CAD build for the part. Positions are in the model's coordinates, mm. A direction names the side the tool comes from. Give positions to 0.01 mm unless a question says otherwise; leave off trailing zeros. Loops run counter-clockwise (first coordinate to the right, second up) from the corner with the lowest first, then second, coordinate; pieces in that order, holes last. Notation, with made-up numbers: (88, 77) -> (131, 77) arc R22 cw to (131, 100) -> close; hole circle Ø2 at (15, 46.25). An arc over 180 degrees is marked (long way). Use one line per item in the form item = value.
```python
from build123d import *

# Parameters (mm, degrees)
SKETCH013_W     = 125.6
SKETCH013_H     = 46.6
PAD007_DEPTH    = 2
CHAMFER_SIZE    = 1.99
SKETCH014_W     = 3.1
SKETCH014_H     = 24
PAD008_DEPTH    = 6
SKETCH015_R     = 1.6
POCKET002_DEPTH = 125.601
SKETCH016_W     = 10
SKETCH016_H     = 3
PAD009_DEPTH    = 14
SKETCH017_R     = 2.2
POCKET003_DEPTH = 5
FILLET001_R     = 4.99
FILLET002_R     = 2.99


with BuildPart() as part:
    # Sketch013 → Pad007 (new body)
    with BuildSketch(Plane.XY.offset(-25)):
        with Locations((0, 1.7)):
            Rectangle(SKETCH013_W, SKETCH013_H)
    extrude(amount=PAD007_DEPTH)

    # Chamfer
    chamfer_edges = [part.edges().sort_by_distance(p)[0] for p in [
        (0, -21.6, -23),
    ]]
    chamfer(chamfer_edges, length=CHAMFER_SIZE)

    # Sketch014 → Pad008 (new body)
    with BuildSketch(Plane.XY.offset(-23)):
        with Locations((-61.25, 7)):
            Rectangle(SKETCH014_W, SKETCH014_H)
    pad008 = extrude(amount=PAD008_DEPTH)

    # Mirrored: Pad008 across Sketch014 V_Axis
    add(pad008.mirror(Plane(origin=(0, 0, -23), x_dir=(0, 0, 1), z_dir=(1, 0, 0))))

    # Sketch015 → Pocket002 (cut, through all)
    with BuildSketch(Plane(origin=(-62.8, 0, -25), x_dir=(0, -1, 0), z_dir=(-1, 0, 0))):
        with Locations((0, 5)):
            Circle(SKETCH015_R)
        with Locations((-14, 5)):
            Circle(SKETCH015_R)
    extrude(amount=-POCKET002_DEPTH, mode=Mode.SUBTRACT)

    # Sketch016 → Pad009 (new body)
    with BuildSketch(Plane.XY.offset(-23)):
        with Locations((-45, 23.5)):
            Rectangle(SKETCH016_W, SKETCH016_H)
        with Locations((45, 23.5)):
            Rectangle(SKETCH016_W, SKETCH016_H)
    extrude(amount=PAD009_DEPTH)

    # Sketch017 → Pocket003 (cut)
    with BuildSketch(Plane(origin=(0, 25, -25), x_dir=(-1, 0, 0), z_dir=(0, 1, 0))):
        with Locations((45, 10)):
            Circle(SKETCH017_R)
    pocket003 = extrude(amount=-POCKET003_DEPTH, mode=Mode.SUBTRACT)

    # Mirrored001: Pocket003 across Sketch017 V_Axis
    add(pocket003.mirror(Plane(origin=(0, 25, -25), x_dir=(0, 1, 0), z_dir=(-1, 0, 0))), mode=Mode.SUBTRACT)

    # Fillet001
    fillet001_edges = [part.edges().sort_by_distance(p)[0] for p in [
        (50, 23.5, -23),
        (50, 23.5, -9),
        (40, 23.5, -9),
        (40, 23.5, -23),
        (-50, 23.5, -23),
        (-50, 23.5, -9),
        (-40, 23.5, -9),
        (-40, 23.5, -23),
    ]]
    fillet(fillet001_edges, radius=FILLET001_R)

    # Fillet002
    fillet002_edges = [part.edges().sort_by_distance(p)[0] for p in [
        (-61.25, 19, -23),
        (-61.25, 19, -17),
        (-61.25, -5, -23),
        (-61.25, -5, -17),
        (61.25, -5, -17),
        (61.25, -5, -23),
        (61.25, 19, -17),
        (61.25, 19, -23),
    ]]
    fillet(fillet002_edges, radius=FILLET002_R)


solid = part.part
```
1. Cut at A-A, the plane y = 14. Write the cut outline in (x, z), then the cut area to 3 significant figures.
Result sheet:
outline = (-62.8, -25) -> (62.8, -25) -> (62.8, -21.6) -> (59.7, -21.6) -> (59.7, -23) -> (-59.7, -23) -> (-59.7, -21.6) -> (-62.8, -21.6) -> close; (-62.8, -18.4) -> (-59.7, -18.4) -> (-59.7, -17) -> (-62.8, -17) -> close; (59.7, -18.4) -> (62.8, -18.4) -> (62.8, -17) -> (59.7, -17) -> close
area = 269 mm^2
2. Cut at D-D, the plane y = -10. Write the cut outline in (x, z).
Result sheet:
outline = (-62.8, -25) -> (62.8, -25) -> (62.8, -23) -> (-62.8, -23) -> close
3. Tool access for faces 4 (the flat face through (-45, 22, -18)), 5 (the flat face through (-50, 23, -16)), 6 (the cylindrical face through (41.423, 23.521, -10.501)): list every direction of +Z, -Z, +X, -X, +Y, -Y with a clear straight run to the whole face (end or side of a thin tool).
Result sheet:
face_4 = +Z, +X, -X, -Y
face_5 = +Z, -X, +Y, -Y
face_6 = +Z, +Y, -Y
4. Cut at B-B, the plane z = -11.25. Write the cut outline in (x, y).
Result sheet:
outline = (-49.18, 22) -> (-40.82, 22) -> (-40.82, 25) -> (-49.18, 25) -> close; (40.82, 22) -> (49.18, 22) -> (49.18, 25) -> (40.82, 25) -> close
5. Mould opens along Z. For faces 1 (the flat face through (-62.8, 7, -22)), 2 (the cylindrical face through (-61.27, 15.18, -18.92)), 3 (the cylindrical face through (61.23, 19.9, -22.15)) say: pulls with the +Z half, pulls with the -Z half, needs draft (parallel to the pull), parting line crosses it, or undercut.
Result sheet:
face_1 = needs draft
face_2 = undercut
face_3 = pulls with the +Z half
6. Drop flat-ended pins along their axis: P1, Ø3.5, axis at y = 23, z = -15.5, coming from the +X side; P2, Ø6, axis at x = 49, z = -11.5, coming from the -Y side; P3, Ø2.5, axis at x = -62, y = 9, coming from the +Z side. Give the stop position or say it passes through.
Result sheet:
P1 = 50
P2 = 22
P3 = -17
7. Drill centre lines: line 1 (Z direction, x = 62, y = 0); line 2 (X direction, y = 7, z = -22.25); line 3 (Z direction, x = 37, y = 12.5). Where is each one in solid material? Low to high.
Result sheet:
line_1 = -25 to -21.6, -18.4 to -17
line_2 = -62.8 to -59.7, 59.7 to 62.8
line_3 = -25 to -23
